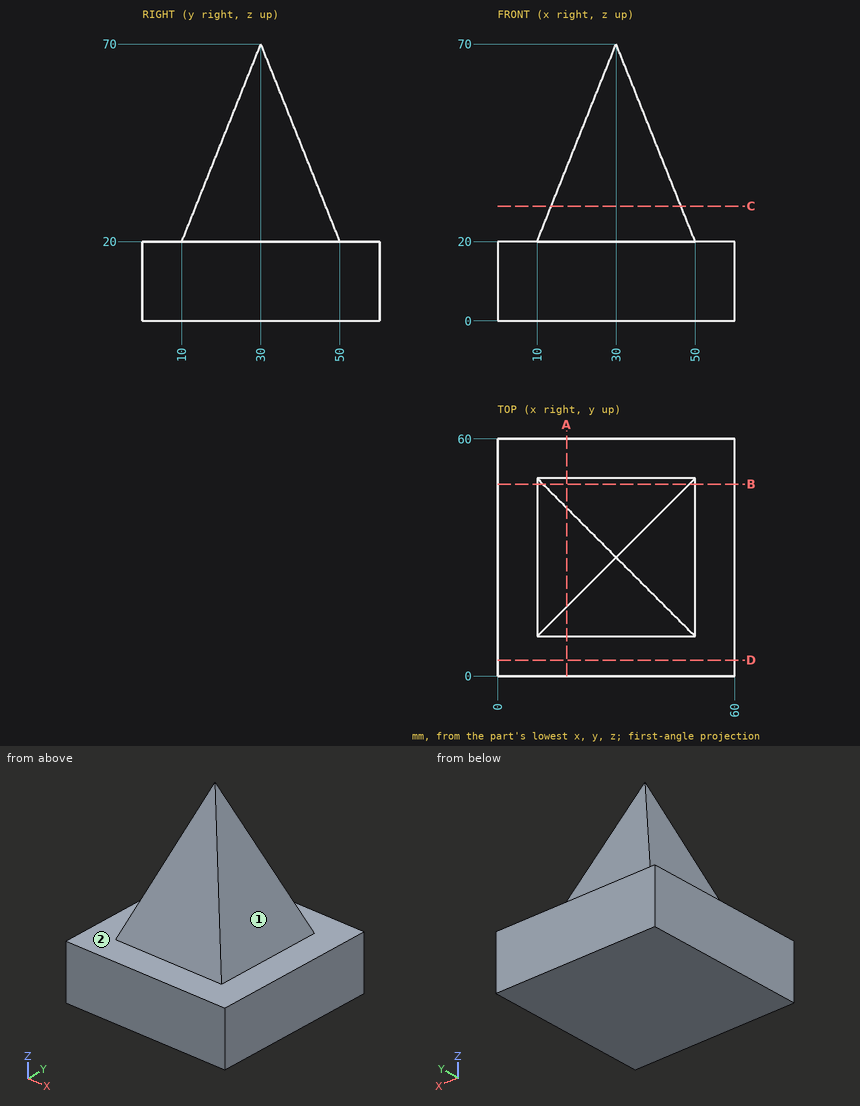
Print and shaded views of the part. All mm, measured from the part's lowest x, y and z. A direction names the side the tool comes from. Coordinates: 2 decimals unless noted, no trailing zeros. Order: outer loops, then holes, each group sorted by start corner. A loop starts at its lowest first (then second) coordinate and runs counter-clockwise, first axis right, second up. Notation, with made-up numbers: M -16.5,61.25 L 24.5,61.25 A9 cw 24.5,69.25 Z; hole C -11.5,-18 d6. An arc over 180 degrees is marked long. One line per question, with ' | ' between items. Start each with the question number.
Q1. Probe L1, parallel to Z at x = 3, y = 33.5; L2, parallel to X at y = 36.5, z = 49.5; L3, parallel to X at y = 34, z = 34. List the from-to ranges inside material, lowest first. Write a range as from..to.
Q2. 3-axis set-ups, long thin cutter, end or side, ignore diameter. For the marked faces 1 and 2: which of +Z, -Z, +X, -X, +Y, -Y reach the whole face in a straight line?
Q3. Flat gauge pins, fed straight in: pin 1 Ø5 at (y, z) = (37, 57) entering from +X; pin 2 Ø8 at (y, z) = (43.5, 30) entering from +X. Where does each tip first touch, or does it go through?
Q4. Saw through at C-C (z = 29). List the corners of the cut face in (x, y).
Q5. Saw through at D-D (y = 4). List the corners of the cut face in (x, z), then the cut area to 3 significant figures.
Q6. Saw through at A-A (x = 17.5). List the corners of the cut face in (y, z), then the cut area to 3 significant figures.
Q7. Saw through at B-B (y = 48.5). List the corners of the cut face in (x, z).
Check values:
1) L1: z = 0..20 | L2: x = 21.8..38.2 | L3: x = 15.6..44.4
2) face 1: +Z, +X, +Y, -Y | face 2: +Z
3) pin 1: stops at x = 36.14 | pin 2: stops at x = 47.6
4) outline: M 13.6,13.6 L 46.4,13.6 L 46.4,46.4 L 13.6,46.4 Z
5) outline: M 0,0 L 60,0 L 60,20 L 0,20 Z | area: 1,200 mm2
6) outline: M 0,0 L 60,0 L 60,20 L 50,20 L 42.5,38.75 L 17.5,38.75 L 10,20 L 0,20 Z | area: 1,810 mm2
7) outline: M 0,0 L 60,0 L 60,20 L 50,20 L 48.5,23.75 L 11.5,23.75 L 10,20 L 0,20 Z
